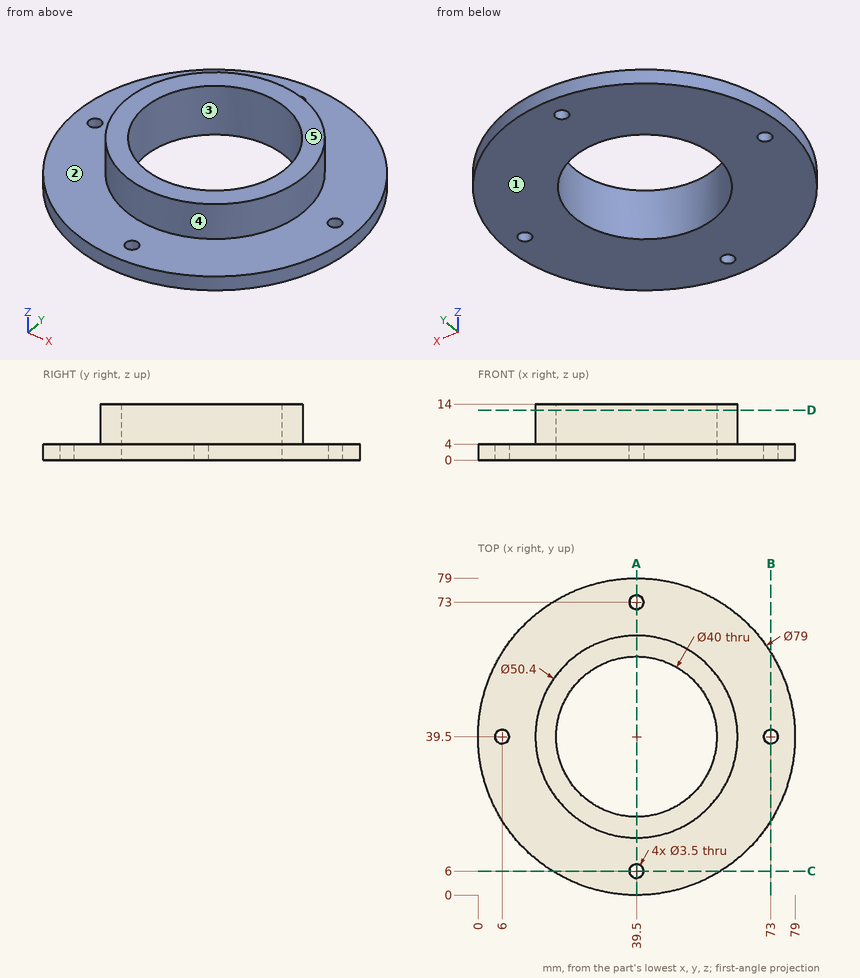
Could you check a few things on this drawing? It's one solid part, dimensions in mm from its lowest x, y, z. A direction names the side the tool comes from. Round coordinates to 2 decimals unless told otherwise and drop trailing zeros. Loops run counter-clockwise (first coordinate to the right, second up) from the corner with the lowest first, then second, coordinate; pieces in that order, holes last.
Q1. Please list where these lines run through material, in increasing order: L1, parallel to Y at x = 39.5, z = 3.25; L2, parallel to Y at x = 39.5, z = 7.25; L3, parallel to Z at x = 8.5, y = 48.
Q2. On a 3-axis mill with a long thin cutter (end or side, diameter ignored), from which of +Z, -Z, +X, -X, +Y, -Y can I reach the whole of each face in a straight line? I mean the marked faces 1 and 2. Say none if no direction works.
Q3. For P1, Ø4, axis at y = 39.5, z = 11.5, coming from the -X side; P2, Ø5, axis at x = 28, y = 25, coming from the +Z side; P3, Ø1.5, axis at x = 20, y = 13, coming from the +Z side; P4, Ø4, axis at y = 63.5, z = 10.5, coming from the +X side, each with a flat end and sliding along its axis, tell me the tip position at first contact or that it passes through.
Q4. I want a section at D-D (z = 12.5). Write out the boundary of the cut face in (x, y).
Q5. I want a section at A-A (x = 39.5). Write out the boundary of the cut face in (y, z), and give its area (3 significant figures).
Q6. I want a section at B-B (x = 73). Write out the boundary of the cut face in (y, z).
Q7. Thinking about a two-plate mould opening in Y: for the marked faces 3, 4 and 5, which applies, pulls with the +Y half, pulls with the -Y half, needs draft (parallel to the pull), parting line crosses it, or undercut?
Answer below:
1. L1: y = 0 to 4.25, 7.75 to 19.5, 59.5 to 71.25, 74.75 to 79
1. L2: y = 14.3 to 19.5, 59.5 to 64.7
1. L3: z = 0 to 4
2. face 1: -Z, +X, -X, +Y, -Y
2. face 2: +Z
3. P1: stops at x = 14.3
3. P2: stops at z = 14
3. P3: stops at z = 4
3. P4: stops at x = 51.79
4. outline: circle Ø50.4 at (39.5, 39.5); hole circle Ø40 at (39.5, 39.5)
5. outline: (0, 0) - (4.25, 0) - (4.25, 4) - (0, 4) - close; (7.75, 0) - (19.5, 0) - (19.5, 14) - (14.3, 14) - (14.3, 4) - (7.75, 4) - close; (59.5, 0) - (71.25, 0) - (71.25, 4) - (64.7, 4) - (64.7, 14) - (59.5, 14) - close; (74.75, 0) - (79, 0) - (79, 4) - (74.75, 4) - close
5. area: 232 mm2
6. outline: (18.57, 0) - (37.75, 0) - (37.75, 4) - (18.57, 4) - close; (41.25, 0) - (60.43, 0) - (60.43, 4) - (41.25, 4) - close
7. face 3: undercut
7. face 4: parting line crosses it
7. face 5: needs draft
